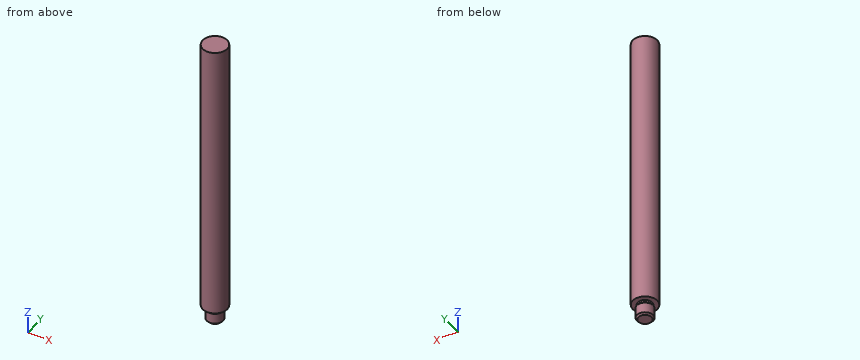
```python
from build123d import *

# Parameters (mm, degrees)
F0_R     = 7.5
F1_DEPTH = 170.5
F2_R     = 5
F3_DEPTH = 9.5
F4_SIZE  = 1


with BuildPart() as f1:
    # F0 (on Top) → F1 (new body)
    with BuildSketch(Plane.XY):
        Circle(F0_R)
    extrude(amount=F1_DEPTH)

    # F2 (on face) → F3 (join)
    with BuildSketch(Plane(origin=(0, 0, 0), x_dir=(1, 0, 0), z_dir=(0, 0, -1))):
        Circle(F2_R)
    extrude(amount=F3_DEPTH)

    # F4
    f4_edges = [f1.edges().sort_by_distance(p)[0] for p in [
        (-5, 0, -9.5),
    ]]
    chamfer(f4_edges, length=F4_SIZE)

    # F5 (on Front) → F6 (revolve, cut)
    with BuildSketch(Plane.XZ):
        Polygon((4.399378, -1.402452), (5.027703, -2.219274), (5.142896, -2.219274), (5.142896, 0), (4.399378, 0), align=None)
    revolve(axis=Axis((0, 0, 0), (0, 0, 1)), mode=Mode.SUBTRACT)


solid = f1.part
```
Design review of the part built by this model. Coordinates are the model's own, in mm. Round coordinates to 2 decimals unless told otherwise and drop trailing zeros. Write each loop counter-clockwise with the first axis right and the second up, starting at its lowest first coordinate (ties: lowest second). Pieces come first, ordered by that corner, then holes. Notation, with made-up numbers: (79, 34) -> (100, 34) arc R30 ccw to (100, 58) -> close; hole circle Ø11 at (-36, 70). An arc over 180 degrees is marked (long way). Answer in a Markdown table with one row per item.
Q1. Take a section at C-C, the plane z = 152.5. State the section outline as (x, y) points.
The answers:
| item | result |
|---|---|
| outline | circle Ø15 at (0, 0) |
Q2. Take a section at A-A, the plane x = 0. State the section outline as (y, z) points, then the cut area to 3 significant figures.
The answers:
| item | result |
|---|---|
| outline | (-7.5, 0) -> (-4.4, 0) -> (-4.4, -1.4) -> (-5, -2.18) -> (-5, -8.5) -> (-4, -9.5) -> (4, -9.5) -> (5, -8.5) -> (5, -2.18) -> (4.4, -1.4) -> (4.4, 0) -> (7.5, 0) -> (7.5, 170.5) -> (-7.5, 170.5) -> close |
| area | 2,650 mm² |
Q3. Clearance check with flat-ended pins moving along their axes: pin 1 Ø1 at (x, y) = (5, -2.5) entering from -Z; pin 2 Ø4 at (y, z) = (4, 111) entering from -X; pin 3 Ø5 at (x, z) = (4, 27.5) entering from +Y. State where each tip first meets the part, or that it passes through.
The answers:
| item | result |
|---|---|
| pin 1 | z = 0 |
| pin 2 | x = -7.23 |
| pin 3 | y = 7.35 |
Q4. To check wall thickness, follow L1, parallel to Z at x = -1.75, y = -5; L2, parallel to Y at x = 0.25, z = 67; L3, parallel to Y at x = 3, z = 104. State the ranges of each line that lie inside material, in increasing order. Write a range as [from, to].
The answers:
| item | result |
|---|---|
| L1 | [0, 170.5] |
| L2 | [-7.5, 7.5] |
| L3 | [-6.87, 6.87] |
